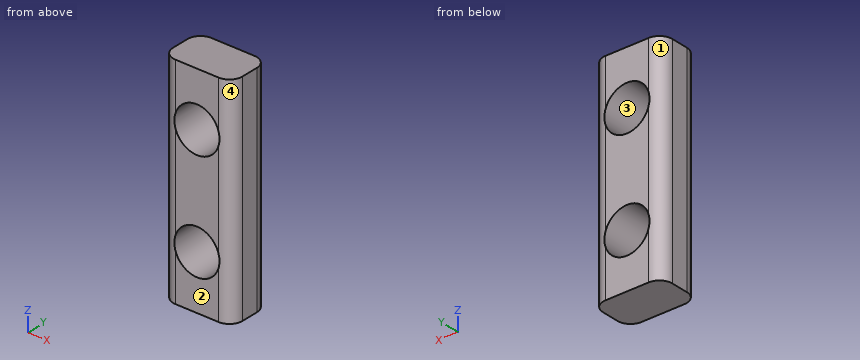
```python
from build123d import *

# Parameters (mm, degrees)
BOSS_EXTRUDE1_DEPTH = 31.75
SKETCH2_R           = 3.302
CUT_EXTRUDE1_DEPTH  = 31.75


with BuildPart() as part:
    # Sketch1 → Boss-Extrude1 (new body)
    with BuildSketch(Plane.XY):
        with BuildLine():
            Line((1.905, 0), (8.255, 0))
            ThreePointArc((8.255, 0), (9.602038418, 0.557961582), (10.16, 1.905))
            Line((10.16, 1.905), (10.16, 4.445))
            ThreePointArc((10.16, 4.445), (9.602038418, 5.792038418), (8.255, 6.35))
            Line((8.255, 6.35), (1.905, 6.35))
            ThreePointArc((1.905, 6.35), (0.557961582, 5.792038418), (0, 4.445))
            Line((0, 4.445), (0, 1.905))
            ThreePointArc((0, 1.905), (0.557961582, 0.557961582), (1.905, 0))
        make_face()
    extrude(amount=BOSS_EXTRUDE1_DEPTH)

    # Sketch2 → Cut-Extrude1 (cut)
    with BuildSketch(Plane(origin=(0, 6.35, 0), x_dir=(1, 0, 0), z_dir=(0, 1, 0))):
        with Locations(Location((5.08, -7.9375, 0), (0, 0, 344.057631394))):
            Circle(SKETCH2_R)
        with Locations(Location((5.08, -23.8125, 0), (0, 0, 344.057631394))):
            Circle(SKETCH2_R)
    extrude(amount=-CUT_EXTRUDE1_DEPTH, mode=Mode.SUBTRACT)


solid = part.part
```
The listing builds one solid part. Answer for the finished solid, in the listing's coordinates (mm). Face numbers are marked on the shaded views. Give positions to 0.01 mm unless a question says otherwise; leave off trailing zeros. Order: outer loops, then holes, each group sorted by start corner. A loop starts at its lowest first (then second) coordinate and runs counter-clockwise, first axis right, second up.
Item 1: The part is cut by section B-B, the plane y = 3. Count the separate pieces of the cut face and the enclosed holes in it, and give its area (3 significant figures).
From the geometry:
separate pieces: 1
enclosed holes: 2
area: 254 mm2
Item 2: The part is cut by section A-A, the plane x = 5.08. Give the vertices of the cut face in (y, z), and give its area (3 significant figures).
From the geometry:
outline: (0, 0) - (6.35, 0) - (6.35, 4.64) - (0, 4.64) - close; (0, 11.24) - (6.35, 11.24) - (6.35, 20.51) - (0, 20.51) - close; (0, 27.11) - (6.35, 27.11) - (6.35, 31.75) - (0, 31.75) - close
area: 118 mm2
Item 3: Find the intervals of material crossed by probe 1 along Z at (x, y) = (5.08, 4.75); probe 2 along Z at (x, y) = (2.25, 4.25); probe 3 along X at (y, z) = (5.5, 23.5), in increasing order.
From the geometry:
probe 1: z = 0 to 4.64, 11.24 to 20.51, 27.11 to 31.75
probe 2: z = 0 to 6.24, 9.64 to 22.11, 25.51 to 31.75
probe 3: x = 0.32 to 1.79, 8.37 to 9.84
Item 4: For a pull along X with two mould halves and no side action, classify the marked faces 1, 2, 3 and 4 as pulls with the +X half, pulls with the -X half, needs draft (parallel to the pull), parting line crosses it, or undercut.
From the geometry:
face 1: pulls with the -X half
face 2: needs draft
face 3: undercut
face 4: pulls with the +X half
Item 5: The part is cut by section D-D, the plane z = 21.5. Give the vertices of the cut face in (x, y) (3 decimals).
From the geometry:
outline: (0, 1.905) arc R1.905 ccw to (1.905, 0) - (2.723, 0) - (2.723, 6.35) - (1.905, 6.35) arc R1.905 ccw to (0, 4.445) - close; (7.437, 0) - (8.255, 0) arc R1.905 ccw to (10.16, 1.905) - (10.16, 4.445) arc R1.905 ccw to (8.255, 6.35) - (7.437, 6.35) - close
Item 6: The part is cut by section C-C, the plane z = 28. Give the vertices of the cut face in (x, y) (3 decimals).
From the geometry:
outline: (0, 1.905) arc R1.905 ccw to (1.905, 0) - (8.255, 0) arc R1.905 ccw to (10.16, 1.905) - (10.16, 4.445) arc R1.905 ccw to (8.255, 6.35) - (1.905, 6.35) arc R1.905 ccw to (0, 4.445) - close
